```python
from build123d import *

# Parameters (mm, degrees)
F1_DEPTH = 10


with BuildPart() as f1:
    # F0 (on Top) → F1 (new body)
    with BuildSketch(Plane.XY):
        with BuildLine():
            ThreePointArc((-114.911513, -3.42815), (-127.747782, -5.627341), (-140.584051, -3.42815))
            ThreePointArc((-140.584051, -3.42815), (-146.385542, -6.834202), (-142.04873, -11.977212))
            Line((-142.04873, -11.977212), (-113.446833, -11.977212))
            ThreePointArc((-113.446833, -11.977212), (-109.110022, -6.834202), (-114.911513, -3.42815))
        make_face()
        with BuildLine():
            Line((-113.446833, -10.977212), (-142.04873, -10.977212))
            ThreePointArc((-142.04873, -10.977212), (-145.399903, -7.003068), (-140.916932, -4.371119))
            ThreePointArc((-140.916932, -4.371119), (-127.747782, -6.627341), (-114.578631, -4.371119))
            ThreePointArc((-114.578631, -4.371119), (-110.095661, -7.003068), (-113.446833, -10.977212))
        make_face(mode=Mode.SUBTRACT)
    extrude(amount=F1_DEPTH)


solid = f1.part
```
Input: part model. Units: mm. Frame: model coordinates. A direction names the side the tool comes from. Coordinates: 2 decimals unless noted, no trailing zeros. Write each loop counter-clockwise with the first axis right and the second up, starting at its lowest first coordinate (ties: lowest second). Pieces come first, ordered by that corner, then holes. Notation, with made-up numbers: (27, 12.5) - (76, 12.5) arc R22 ccw to (76, 19.5) - close; hole circle Ø4 at (9, -15). An arc over 180 degrees is marked (long way). Put each result on its own line as item: value. Start each with the question number.
1) Reachability of faces 4 (the face through (-127.565, -5.627, 4.93)), 5 (the face through (-128, -10.977, 5)) from +Z, -Z, +X, -X, +Y, -Y: full face, straight path, thin tool, end or side. Return the list, or none.
2) Mould query, pull axis Y, two halves, no side actions, for faces 1 (the face through (-110.11, -6.92, 4.93)), 2 (the face through (-109.1, -6.9, 4.9)), 3 (the face through (-128, -6, 10)). Classes: pulls with the +Y half, pulls with the -Y half, needs draft (parallel to the pull), parting line crosses it, or undercut.
3) Ray query, L1, parallel to X at y = -7.5, z = 7; L2, parallel to Y at x = -117, z = 4; L3, parallel to Y at x = -140.5, z = 3.5. Return the intervals inside material, ascending.
4) Contact query for flat-ended pins moving along their axis: pin 1 (4 mm diameter, centred on y = -5.5, z = 7, fed in from +X); pin 2 (1.5 mm diameter, centred on x = -135, z = 7, fed in from +Y); pin 3 (4 mm diameter, centred on y = -4, z = 3.5, fed in from +X); pin 4 (5 mm diameter, centred on y = -4, z = 6, fed in from -X). Output: stop coordinate, or through.
5) Cut plane D-D (y = -10). Return the cut outline in (x, z).
6) Cut plane C-C (x = -125). Return the cut outline in (y, z), plus the area to 3 significant figures.
7) Cut plane A-A (z = 3). Return the cut outline in (x, y), plus the area to 3 significant figures.
8) Cut plane B-B (y = -5). Return the cut outline in (x, z), plus the area to 3 significant figures.
Resolved:
1. face 4: +Z, -Z, +Y
1. face 5: +Z, -Z
2. face 1: undercut
2. face 2: parting line crosses it
2. face 3: needs draft
3. L1: x = -146.45 to -145.45, -110.05 to -109.05
3. L2: y = -11.98 to -10.98, -5.14 to -4.1
3. L3: y = -11.98 to -10.98, -4.52 to -3.46
4. pin 1: stops at x = -109.05
4. pin 2: stops at y = -4.79
4. pin 3: stops at x = -109.34
4. pin 4: stops at x = -146.31
5. outline: (-145.72, 0) - (-144.43, 0) - (-144.43, 10) - (-145.72, 10) - close; (-111.06, 0) - (-109.77, 0) - (-109.77, 10) - (-111.06, 10) - close
6. outline: (-11.98, 0) - (-10.98, 0) - (-10.98, 10) - (-11.98, 10) - close; (-6.53, 0) - (-5.53, 0) - (-5.53, 10) - (-6.53, 10) - close
6. area: 20.0 mm2
7. outline: (-142.05, -11.98) - (-113.45, -11.98) arc R4.4 ccw (long way) to (-114.91, -3.43) arc R38.56 cw to (-140.58, -3.43) arc R4.4 ccw (long way) to start; hole (-142.05, -10.98) - (-113.45, -10.98) arc R3.4 ccw (long way) to (-114.58, -4.37) arc R39.56 cw to (-140.92, -4.37) arc R3.4 ccw (long way) to start
7. area: 82.3 mm2
8. outline: (-145.61, 0) - (-144.27, 0) - (-144.27, 10) - (-145.61, 10) - close; (-138.98, 0) - (-134.68, 0) - (-134.68, 10) - (-138.98, 10) - close; (-120.82, 0) - (-116.52, 0) - (-116.52, 10) - (-120.82, 10) - close; (-111.23, 0) - (-109.88, 0) - (-109.88, 10) - (-111.23, 10) - close
8. area: 113 mm2
